```python
from build123d import *

# Parameters (mm, degrees)
F0_W     = 101.6
F0_H     = 63.5
F1_DEPTH = 25.4
F2_R     = 6.35
F3_DEPTH = 25.401
F4_W     = 12.7
F4_H     = 25.4
F6_W     = 13.615308
F6_H     = 6.35


with BuildPart() as f1:
    # F0 (on Top) → F1 (new body)
    with BuildSketch(Plane.XY):
        Rectangle(F0_W, F0_H)
    extrude(amount=F1_DEPTH)

    # F2 (on face) → F3 (cut, through all)
    with BuildSketch(Plane.XY.offset(25.4)):
        with Locations((-38.1, 19.05)):
            Circle(F2_R)
        with Locations((38.1, 19.05)):
            Circle(F2_R)
        with Locations((38.1, -19.05)):
            Circle(F2_R)
        with Locations((-38.1, -19.05)):
            Circle(F2_R)
    extrude(amount=-F3_DEPTH, mode=Mode.SUBTRACT)

    # F4 (on Front) → F5 (revolve)
    with BuildSketch(Plane.XZ):
        with Locations((-6.35, 38.1)):
            Rectangle(F4_W, F4_H)
    revolve(axis=Axis((0, 0, 38.1), (0, 0, 1)))

    # F6 (on Front) → F7 (revolve, cut)
    with BuildSketch(Plane.XZ):
        with Locations((-14.427654, 34.925)):
            Rectangle(F6_W, F6_H)
    revolve(axis=Axis((0, 0, 50.8), (0, 0, 1)), mode=Mode.SUBTRACT)


solid = f1.part
```
Here's how the part is built. I have some questions about the finished solid (model axes, mm). A direction names the side the tool comes from. Give positions to 0.01 mm unless a question says otherwise; leave off trailing zeros. Order: outer loops, then holes, each group sorted by start corner. A loop starts at its lowest first (then second) coordinate and runs counter-clockwise, first axis right, second up. Notation, with made-up numbers: (-12.75, -21) - (15.25, -21) arc R30 cw to (15.25, 14) - close; hole circle Ø4 at (-22.75, -30). An arc over 180 degrees is marked (long way). Answer as a JSON object with one key per item and string values. Group by question number.
Item 1: Please list where these lines run through material, in increasing order: probe 1 along X at (y, z) = (19, 16); probe 2 along Y at (x, z) = (-38.1, 6); probe 3 along Z at (x, y) = (-7, 7.5).
Item 2: If we section it at C-C on z = 16.5: Please give me the cut outline in (x, y).
Item 3: If we section it at B-B on x = 38.1: Please give me the cut outline in (y, z).
Item 4: If we section it at D-D on x = -11.5: Please give me the cut outline in (y, z).
Item 5: If we mould it in two halves opening along Z, with no side actions, what happens to faces 4 (the cylindrical face through (1.65, 7.44, 34.97)), 5 (the flat face through (-5.5, 5.5, 31.75)), 6 (the cylindrical face through (-32.043, 20.957, 12.878)), 7 (the flat face through (-1, 0, 0))? For each: pulls with the +Z half, pulls with the -Z half, needs draft (parallel to the pull), parting line crosses it, or undercut.
Item 6: If we section it at A-A on y = -19.05: Please give me the cut outline in (x, z), and give its area (3 significant figures).
Item 7: For P1, Ø8, axis at x = 39.5, y = 14, coming from the -Z side; P2, Ø19, axis at x = 22, y = -15.5, coming from the +Z side; P3, Ø12, axis at y = -6.5, z = 45, coming from the +X side, each with a flat end and sliding along its axis, tell me the tip position at first contact or that it passes through.
Item 8: Which directions (+Z, -Z, +X, -X, +Y, -Y) give clear straight access to the entire face, cutting with the end or side of a thin tool? Please do faces 1 (the flat face through (-5.5, 5.5, 38.1)), 2 (the flat face through (-50.8, 0, 13)), 3 (the cylindrical face through (2.75, 12.4, 44.54)).
Result set:
{
 "1": {"probe 1": "-50.8 to -44.45, -31.75 to 31.75, 44.45 to 50.8", "probe 2": "-31.75 to -25.4, -12.7 to 12.7, 25.4 to 31.75", "probe 3": "0 to 31.75, 38.1 to 50.8"},
 "2": {"outline": "(-50.8, -31.75) - (50.8, -31.75) - (50.8, 31.75) - (-50.8, 31.75) - close; hole circle Ø12.7 at (-38.1, -19.05); hole circle Ø12.7 at (-38.1, 19.05); hole circle Ø12.7 at (38.1, -19.05); hole circle Ø12.7 at (38.1, 19.05)"},
 "3": {"outline": "(-31.75, 0) - (-25.4, 0) - (-25.4, 25.4) - (-31.75, 25.4) - close; (-12.7, 0) - (12.7, 0) - (12.7, 25.4) - (-12.7, 25.4) - close; (25.4, 0) - (31.75, 0) - (31.75, 25.4) - (25.4, 25.4) - close"},
 "4": {"outline": "(-31.75, 0) - (31.75, 0) - (31.75, 25.4) - (5.39, 25.4) - (5.39, 31.75) - (-5.39, 31.75) - (-5.39, 25.4) - (-31.75, 25.4) - close; (-5.39, 38.1) - (5.39, 38.1) - (5.39, 50.8) - (-5.39, 50.8) - close"},
 "5": {"face 4": "undercut", "face 5": "undercut", "face 6": "needs draft", "face 7": "pulls with the -Z half"},
 "6": {"outline": "(-50.8, 0) - (-44.45, 0) - (-44.45, 25.4) - (-50.8, 25.4) - close; (-31.75, 0) - (31.75, 0) - (31.75, 25.4) - (-31.75, 25.4) - close; (44.45, 0) - (50.8, 0) - (50.8, 25.4) - (44.45, 25.4) - close", "area": "1,940 mm²"},
 "7": {"P1": "z = 0", "P2": "z = 25.4", "P3": "x = 12.69"},
 "8": {"face 1": "none", "face 2": "+Z, -Z, -X, +Y, -Y", "face 3": "+Z"}
}
